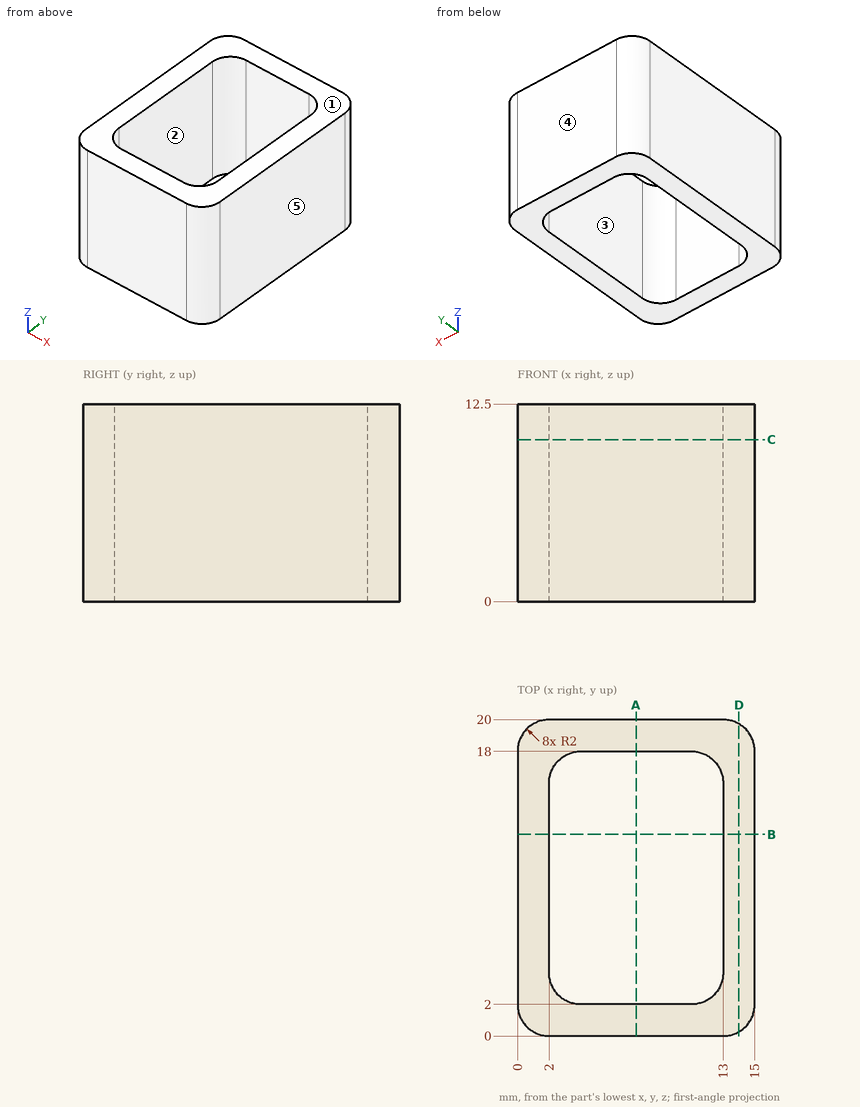
Source: three-view drawing plus pictorial views. Frame: mm from the lowest corner of the part. A direction names the side the tool comes from. Round coordinates to 2 decimals unless told otherwise and drop trailing zeros. Loops run counter-clockwise (first coordinate to the right, second up) from the corner with the lowest first, then second, coordinate; pieces in that order, holes last.
1. Mould query, pull axis X, two halves, no side actions, for the marked faces 3, 4 and 5. Classes: released by +X, released by -X, zero draft, split by the parting line, or undercut.
2. Contact query for a flat-ended pin moving along its axis: pin 1 (2 mm diameter, centred on x = 13, y = 18, fed in from -Z). Output: stop coordinate, or through.
3. Section query D-D on x = 14. Output: boundary loops of the cut face in (y, z).
4. Section query C-C on z = 10.25. Output: boundary loops of the cut face in (x, y).
5. Access query for the marked faces 1 and 2. Directions: +Z, -Z, +X, -X, +Y, -Y. A direction counts if a zero-diameter tool reaches every point of the face in a straight line with its end or side. Return the directions, or none.
6. Ray query, L1, parallel to X at y = 12, z = 2; L2, parallel to Y at x = 5, z = 5.5; L3, parallel to X at y = 3, z = 11. Return the intervals inside material, ascending.
7. Section query A-A on x = 7.5. Output: boundary loops of the cut face in (y, z).
8. Section query B-B on y = 12.75. Output: boundary loops of the cut face in (x, z).
Answers below:
1. face 3: undercut
1. face 4: zero draft
1. face 5: released by +X
2. pin 1: stops at z = 0
3. outline: (0.27, 0) - (19.73, 0) - (19.73, 12.5) - (0.27, 12.5) - close
4. outline: (0, 2) arc R2 ccw to (2, 0) - (13, 0) arc R2 ccw to (15, 2) - (15, 18) arc R2 ccw to (13, 20) - (2, 20) arc R2 ccw to (0, 18) - close; hole (2, 4) arc R2 ccw to (4, 2) - (11, 2) arc R2 ccw to (13, 4) - (13, 16) arc R2 ccw to (11, 18) - (4, 18) arc R2 ccw to (2, 16) - close
5. face 1: +Z, +X, -X, +Y, -Y
5. face 2: +Z, -Z
6. L1: x = 0 to 2, 13 to 15
6. L2: y = 0 to 2, 18 to 20
6. L3: x = 0 to 2.27, 12.73 to 15
7. outline: (0, 0) - (2, 0) - (2, 12.5) - (0, 12.5) - close; (18, 0) - (20, 0) - (20, 12.5) - (18, 12.5) - close
8. outline: (0, 0) - (2, 0) - (2, 12.5) - (0, 12.5) - close; (13, 0) - (15, 0) - (15, 12.5) - (13, 12.5) - close
